Verification items for the finished model (mm, model axes). A direction names the side the tool comes from. Give positions to 0.01 mm unless a question says otherwise; leave off trailing zeros. Loops run counter-clockwise (first coordinate to the right, second up) from the corner with the lowest first, then second, coordinate; pieces in that order, holes last. Notation, with made-up numbers: (-6, 16) - (18, 16) arc R13 ccw to (18, 41) - close; hole circle Ø8 at (40.5, 44.25). An arc over 180 degrees is marked (long way). Use one line per item in the form item = value.
Autodesk Inventor part; units mm, degrees
ref_plane "Work Plane1" through (0, 0, 5) normal (0, 0, 1) x (1, 0, 0)
ref_plane "YZ Plane" through (0, 0, 0) normal (1, 0, 0) x (0, 1, 0)
ref_plane "XZ Plane" through (0, 0, 0) normal (0, 1, 0) x (-1, 0, 0)
sketch "Sketch1" plane through (0, 0, 0) normal (0, 0, 1) x (1, 0, 0)
  line L0 (0, 0) -> (50.8, 0)
  line L1 (50.8, 0) -> (50.8, 10)
  line L2 (0, 10) -> (0, 0)
  circle A0 centre (8.25, 30) radius 4.875
  arc A1 (16.5, 30) -> (0, 30) centre (8.25, 30) ccw
  line L3 (25.4, -5.1734) -> (25.4, 32.937)
  line L4 (0, 30) -> (0, 10)
  line L5 (16.5, 30) -> (16.5, 10)
  line L6 (50.8, 10) -> (16.5, 10)
  line L7 (0, 10) -> (0, 10)
  circle A2 centre (42.55, 30) radius 4.875
  arc A3 (50.8, 30) -> (34.3, 30) centre (42.55, 30) ccw
  line L8 (50.8, 30) -> (50.8, 10)
  line L9 (34.3, 30) -> (34.3, 10)
  line L10 (-14.5687, 38) -> (58.8919, 38)
  line L11 (58.8919, 38) -> (58.8919, 91.2703)
  line L12 (58.8919, 91.2703) -> (-14.5687, 91.2703)
  line L13 (-14.5687, 91.2703) -> (-14.5687, 38)
  point P0 (25.4, 0)
  point P1 (34.3, 10)
  point P2 (44.5656, 38)
  point P3 (40.5344, 38)
  point P4 (10.2656, 38)
  point P5 (6.2344, 38)
  dimension "d0" = 0
  dimension "d1" = 50.8
  dimension "d2" = 8.25
  dimension "d3" = 9.75
  dimension "d4" = 16.5
  dimension "d7" = 10
  dimension "d8" = 0
  dimension "d19" = 20
  dimension "d21" = 28
extrude "Extrusion1" add sketch "Sketch1" along normal blind 10 contours L2 L4 A1 L10 L5 L6 L3 L0 | L3 L6 L1 L0 | L6 L9 A3 L10 L8
ref_plane "Work Plane1" through (0, 0, 5) normal (0, 0, 1) x (1, 0, 0)
sketch "Sketch2" plane through (0, 0, 5) normal (0, 0, 1) x (1, 0, 0)
  line L0 (0, 0) -> (50.8, 0)
  line L1 (50.8, 0) -> (50.8, 30)
  arc A0 (50.8, 30) -> (44.5656, 38) centre (42.55, 30) ccw
  line L2 (34.3, 30) -> (34.3, 10)
  line L3 (34.3, 10) -> (16.5, 10)
  line L4 (16.5, 10) -> (16.5, 30)
  arc A1 (16.5, 30) -> (10.2656, 38) centre (8.25, 30) ccw
  line L5 (0, 30) -> (0, 0)
  circle A2 centre (42.55, 30) radius 4.875
  circle A3 centre (8.25, 30) radius 4.875
  line L6 (0, 0) -> (5, 0)
  line L7 (5, 0) -> (5, 10)
  line L8 (5, 10) -> (0, 10)
  line L9 (0, 10) -> (0, 0)
  line L10 (50.8, 0) -> (45.8, 0)
  line L11 (45.8, 0) -> (45.8, 10)
  line L12 (45.8, 10) -> (50.8, 10)
  line L13 (50.8, 10) -> (50.8, 0)
  line L14 (44.5656, 38) -> (40.5344, 38)
  arc A4 (40.5344, 38) -> (34.3, 30) centre (42.55, 30) ccw
  line L15 (10.2656, 38) -> (6.2344, 38)
  arc A5 (6.2344, 38) -> (0, 30) centre (8.25, 30) ccw
  dimension "d10" = 5
  dimension "d11" = 5
  dimension "d12" = 10
  dimension "d13" = 10
extrude "Extrusion2" add sketch "Sketch2" along normal mid plane 40 contours L5 L8 L7 L0 | L11 L12 L1 L0
chamfer "Chamfer1" distance 5 angle 45 4 edges at (2.5, 10, 25) (48.3, 10, 25) (48.3, 10, -15) (2.5, 10, -15)
equation "\"d2\" = 0.5 * Platform_GuideRod_OD"
equation "\"d4\" = Platform_GuideRod_OD"
equation "\"d7\" = Thick_Wall"
equation "\"d21\" = Sliding_Clearance + Actuator_Housing_W"
equation "\"d5\" = Thick_Wall"
equation "\"d11\" = d10"
equation "\"d12\" = Thick_Wall"
equation "\"d13\" = d12"
equation "\"d16\" = 0.5 * Thick_Wall"
equation "\"Platform_Width\" = 50.8"
equation "\"Platform_Length\" = 245"
equation "\"Guide_Hole_Offset\" = 13.51"
equation "\"Guide_Rod_Diameter\" = 6"
equation "\"Guide_Rod_Length\" = 304.8"
equation "\"Thin_Wall\" = 5"
equation "\"Thick_Wall\" = 10"
equation "\"Tabletop_Hole_Spacing\" = 25.4"
equation "\"Tabletop_Hole_Diameter\" = 6.35"
equation "\"Platform_Hole_Spacing\" = 25.4"
equation "\"Platform_Hole_Diameter\" = 6.35"
equation "\"Actuator_Housing_W\" = 26"
equation "\"Sliding_Clearance\" = 2"
equation "\"Platform_GuideRod_OD\" = 16.5"
equation "\"d9\" = -0.5 * Thick_Wall"
properties part number "Guide Rod Support"
1. Section check A-A, the plane y = 22. Record the cut outline in (x, z).
Result set:
outline = (0, 0) - (16.5, 0) - (16.5, 10) - (0, 10) - close; (34.3, 0) - (50.8, 0) - (50.8, 10) - (34.3, 10) - close
2. Tool access check on faces 1 (the flat face through (48, 10, -5)), 2 (the cylindrical face through (14.71, 35.13, 4.93)), 3 (the flat face through (45.8, 5, -8)). Record the directions out of +Z, -Z, +X, -X, +Y, -Y that give a thin tool (end or side, any length) a straight path to the whole face; none if there is none.
Result set:
face_1 = -Z, +X, -X, +Y
face_2 = +Z, -Z, +Y
face_3 = -Z, +Y, -Y
3. Section check D-D, the plane y = 32.5. Record the cut outline in (x, z).
Result set:
outline = (0.39, 0) - (4.06, 0) - (4.06, 10) - (0.39, 10) - close; (12.44, 0) - (16.11, 0) - (16.11, 10) - (12.44, 10) - close; (34.69, 0) - (38.36, 0) - (38.36, 10) - (34.69, 10) - close; (46.74, 0) - (50.41, 0) - (50.41, 10) - (46.74, 10) - close
4. Section check B-B, the plane x = 42.55. Record the cut outline in (y, z) (3 decimals), then the cut area to 4 significant figures.
Result set:
outline = (0, 0) - (25.125, 0) - (25.125, 10) - (0, 10) - close; (34.875, 0) - (38, 0) - (38, 10) - (34.875, 10) - close
area = 282.5 mm²
5. Draft check along Y on faces 4 (the flat face through (8, 38, 5)), 5 (the flat face through (16.5, 20, 5)), 6 (the cylindrical face through (38.681, 32.966, 4.93)). Enter one of: released by +Y, released by -Y, zero draft, split by the parting line, or undercut.
Result set:
face_4 = released by +Y
face_5 = zero draft
face_6 = undercut
6. Scan lines: probe 1 along Y at (x, z) = (42.55, 3) (3 decimals); probe 2 along X at (y, z) = (4, -7); probe 3 along Z at (x, y) = (34.5, 30). Record each from-to range of solid material in increasing order.
Result set:
probe_1 = 0 to 25.125, 34.875 to 38
probe_2 = 0 to 5, 45.8 to 50.8
probe_3 = 0 to 10
7. Depth check by flat-ended pin: pin 1 Ø15.5 at (x, y) = (8.25, 30) entering from +Z; pin 2 Ø2.5 at (x, z) = (1.5, 13.5) entering from +Y; pin 3 Ø19 at (x, y) = (25, 22.5) entering from -Z. Enter the tip coordinate at first touch or a pass-through.
Result set:
pin_1 = 10
pin_2 = 10
pin_3 = 0
8. Section check C-C, the plane z = 4. Record the cut outline in (x, y) (3 decimals), then the cut area to 3 significant figures.
Result set:
outline = (0, 0) - (50.8, 0) - (50.8, 30) arc R8.25 ccw to (44.566, 38) - (40.534, 38) arc R8.25 ccw to (34.3, 30) - (34.3, 10) - (16.5, 10) - (16.5, 30) arc R8.25 ccw to (10.266, 38) - (6.234, 38) arc R8.25 ccw to (0, 30) - close; hole circle Ø9.75 at (8.25, 30); hole circle Ø9.75 at (42.55, 30)
area = 1,230 mm²
